```python
from build123d import *

# Parameters (mm, degrees)
SKETCH1_R           = 3.5
BOSS_EXTRUDE1_DEPTH = 4
SKETCH2_R           = 2
BOSS_EXTRUDE2_DEPTH = 1
CUT_EXTRUDE1_DEPTH  = 3


with BuildPart() as part:
    # Sketch1 → Boss-Extrude1 (new body)
    with BuildSketch(Plane(origin=(0, 0, 0), x_dir=(1, 0, 0), z_dir=(0, 1, 0))):
        Circle(SKETCH1_R)
    extrude(amount=BOSS_EXTRUDE1_DEPTH)

    # Sketch2 → Boss-Extrude2 (add)
    with BuildSketch(Plane.XZ):
        Circle(SKETCH2_R)
    extrude(amount=BOSS_EXTRUDE2_DEPTH)

    # Sketch3 → Cut-Extrude1 (cut)
    with BuildSketch(Plane(origin=(0, 4, 0), x_dir=(1, 0, 0), z_dir=(0, 1, 0))):
        Polygon((1.732050808, 0), (0.866025404, 1.5), (-0.866025404, 1.5), (-1.732050808, 0), (-0.866025404, -1.5), (0.866025404, -1.5), align=None)
    extrude(amount=-CUT_EXTRUDE1_DEPTH, mode=Mode.SUBTRACT)


solid = part.part
```
Can you work these out from the model? Positions are in its coordinate system, mm. A direction names the side the tool comes from. Give positions to 0.01 mm unless a question says otherwise; leave off trailing zeros. Loops run counter-clockwise (first coordinate to the right, second up) from the corner with the lowest first, then second, coordinate; pieces in that order, holes last. Notation, with made-up numbers: M -4.75,41 L 9.25,41 A24 cw 9.25,74 Z; hole C 73.5,27 d11. An arc over 180 degrees is marked long. Use CSV: the item, a comma, the result in double quotes. Start each with the question number.
1. On a 3-axis mill with a long thin cutter (end or side, diameter ignored), from which of +Z, -Z, +X, -X, +Y, -Y can I reach the whole of each face in a straight line? I mean faces 1 (the face through (2, 0, 2)), 2 (the face through (0, 4, 2)), 3 (the face through (0, 3, 1.5)). Say none if no direction works.
2. If we mould it in two halves opening along X, with no side actions, what happens to faces 4 (the face through (0, -1, 0)), 5 (the face through (1.305, 2.521, -0.74)), 6 (the face through (3.233, 1.972, 1.341))? For each: released by +X, released by -X, zero draft, split by the parting line, or undercut.
3. For P1, Ø3, axis at y = 1, z = 2, coming from the -X side; P2, Ø3, axis at x = -2, y = 0.5, coming from the +Z side, each with a flat end and sliding along its axis, tell me the tip position at first contact or that it passes through.
4. Imagine slicing it at C-C, the plane z = -1. Write out the boundary of the cut face in (x, y).
5. Imagine slicing it at A-A, the plane y = 1.1. Write out the boundary of the cut face in (x, z), plus the area to 3 significant figures.
6. Imagine slicing it at B-B, the plane x = 0. Write out the boundary of the cut face in (y, z).
7. Imagine slicing it at D-D, the plane x = -2.5. Write out the boundary of the cut face in (y, z), plus the area to 3 significant figures.
8. If I drill on L1, parallel to Z at x = 0, y = 3.8; L2, parallel to Y at x = -2, z = -0.75; L3, parallel to Y at x = -0.25, z = -1.25, over which ranges is the centre line in solid material (lowest first)?
Response values:
1,face 1,"-Y"
1,face 2,"+Z, -Z, +X, -X, +Y"
1,face 3,"+Y"
2,face 4,"zero draft"
2,face 5,"undercut"
2,face 6,"split by the parting line"
3,P1,"x = -3.46"
3,P2,"z = 3.46"
4,outline,"M -3.35,0 L -1.73,0 L -1.73,-1 L 1.73,-1 L 1.73,0 L 3.35,0 L 3.35,4 L 1.15,4 L 1.15,1 L -1.15,1 L -1.15,4 L -3.35,4 Z"
5,outline,"C 0,0 d7; hole M -1.73,0 L -0.87,-1.5 L 0.87,-1.5 L 1.73,0 L 0.87,1.5 L -0.87,1.5 Z"
5,area,"30.7 mm^2"
6,outline,"M -1,-2 L 0,-2 L 0,-3.5 L 4,-3.5 L 4,-1.5 L 1,-1.5 L 1,1.5 L 4,1.5 L 4,3.5 L 0,3.5 L 0,2 L -1,2 Z"
7,outline,"M 0,-2.45 L 4,-2.45 L 4,2.45 L 0,2.45 Z"
7,area,"19.6 mm^2"
8,L1,"-3.5 to -1.5, 1.5 to 3.5"
8,L2,"0 to 4"
8,L3,"-1 to 1"
